Geometry: final body of the model. Coordinates: model frame, mm. A direction names the side the tool comes from. Give positions to 0.01 mm unless a question says otherwise; leave off trailing zeros. Loops run counter-clockwise (first coordinate to the right, second up) from the corner with the lowest first, then second, coordinate; pieces in that order, holes last.
from build123d import *

# Parameters (mm, degrees)
BOX003_W     = 4.9
BOX003_H     = 12.4
BOX003_DEPTH = 20
BOX002_W     = 4.9
BOX002_H     = 12.4
BOX002_DEPTH = 20
BOX001_W     = 4.9
BOX001_H     = 12.4
BOX001_DEPTH = 20
BOX_W        = 52
BOX_H        = 20
BOX_DEPTH    = 15


with BuildPart() as slot003:
    # Box003 → Box003 (new body)
    with BuildSketch(Plane(origin=(43.5, 3.5, 4), x_dir=(1, 0, 0), z_dir=(0, 0, 1))):
        with Locations((2.45, 6.2)):
            Rectangle(BOX003_W, BOX003_H)
    extrude(amount=BOX003_DEPTH)


with BuildPart() as slot002:
    # Box002 → Box002 (new body)
    with BuildSketch(Plane(origin=(23.5, 3.5, 4), x_dir=(1, 0, 0), z_dir=(0, 0, 1))):
        with Locations((2.45, 6.2)):
            Rectangle(BOX002_W, BOX002_H)
    extrude(amount=BOX002_DEPTH)


with BuildPart() as slots:
    # Box001 → Box001 (new body)
    with BuildSketch(Plane(origin=(3.5, 3.5, 4), x_dir=(1, 0, 0), z_dir=(0, 0, 1))):
        with Locations((2.45, 6.2)):
            Rectangle(BOX001_W, BOX001_H)
    extrude(amount=BOX001_DEPTH)

    # Fusion: union slot003, slot002
    add(slot003.part)
    add(slot002.part)


with BuildPart() as obj1:
    # Box → Box (new body)
    with BuildSketch(Plane.XY):
        with Locations((26, 10)):
            Rectangle(BOX_W, BOX_H)
    extrude(amount=BOX_DEPTH)

    # Cut: cut slots
    add(slots.part, mode=Mode.SUBTRACT)


solid = obj1.part
Item 1: Draft query along X for faces 3 (the face through (31, 10, 15)), 4 (the face through (3.5, 10, 9)), 5 (the face through (0, 10, 7)). Return one class per face: +X half, -X half, draft (parallel to the pull), parting line (faces both ways), or undercut.
Values follow:
face 3: draft
face 4: undercut
face 5: -X half
Item 2: Ray query, probe 1 along X at (y, z) = (5, 5); probe 2 along Y at (x, z) = (25, 10.5); probe 3 along Z at (x, y) = (28, 4.5). Return the intervals inside material, ascending.
Values follow:
probe 1: x = 0 to 3.5, 8.4 to 23.5, 28.4 to 43.5, 48.4 to 52
probe 2: y = 0 to 3.5, 15.9 to 20
probe 3: z = 0 to 4
Item 3: Pin query (flat end, axial travel): pin 1 (5.5 mm diameter, centred on x = 25, z = 8.5, fed in from -Y); pin 2 (1.5 mm diameter, centred on x = 47, y = 11.5, fed in from +Z). Return the tip coordinate at first contact, or that it passes through.
Values follow:
pin 1: stops at y = 0
pin 2: stops at z = 4
Item 4: Section query B-B on x = 44.5. Return loops of the section in (y, z), plus the area to 3 significant figures.
Values follow:
outline: (0, 0) - (20, 0) - (20, 15) - (15.9, 15) - (15.9, 4) - (3.5, 4) - (3.5, 15) - (0, 15) - close
area: 164 mm2
Item 5: Section query A-A on z = 12.5. Return loops of the section in (x, y).
Values follow:
outline: (0, 0) - (52, 0) - (52, 20) - (0, 20) - close; hole (3.5, 3.5) - (8.4, 3.5) - (8.4, 15.9) - (3.5, 15.9) - close; hole (23.5, 3.5) - (28.4, 3.5) - (28.4, 15.9) - (23.5, 15.9) - close; hole (43.5, 3.5) - (48.4, 3.5) - (48.4, 15.9) - (43.5, 15.9) - close
Item 6: Section query C-C on y = 8.5. Return loops of the section in (x, z), plus the area to 3 significant figures.
Values follow:
outline: (0, 0) - (52, 0) - (52, 15) - (48.4, 15) - (48.4, 4) - (43.5, 4) - (43.5, 15) - (28.4, 15) - (28.4, 4) - (23.5, 4) - (23.5, 15) - (8.4, 15) - (8.4, 4) - (3.5, 4) - (3.5, 15) - (0, 15) - close
area: 618 mm2
Item 7: Set-up query: faces 1 (the face through (26, 15.9, 9)), 2 (the face through (26, 20, 7)). Return all of +Z, -Z, +X, -X, +Y, -Y with unobstructed straight access to the full face (end or side cutting, diameter ignored); none if empty.
Values follow:
face 1: +Z
face 2: +Z, -Z, +X, -X, +Y
